from build123d import *

# Parameters (mm, degrees)
F0_R     = 10.16
F1_DEPTH = 76.2
F3_DEPTH = 27.94
F5_DEPTH = 10.16
F6_R     = 7.62
F7_DEPTH = 10.16
F8_R     = 10.16


with BuildPart() as f1:
    # F0 (on Front) → F1 (new body)
    with BuildSketch(Plane.XZ):
        Polygon((-96.203486, 15.24), (-96.203486, -20.32), (15.556514, -20.32), (51.116514, 15.24), (51.116514, 50.8), (15.556514, 50.8), (-20.003486, 15.24), align=None)
        Circle(F0_R, mode=Mode.SUBTRACT)
    extrude(amount=-F1_DEPTH)

    # F2 (on face) → F3 (cut)
    with BuildSketch(Plane.XY.offset(50.8)):
        with BuildLine():
            ThreePointArc((25.716514, 15.24), (33.336514, 7.62), (40.956514, 15.24))
            Line((40.956514, 15.24), (40.956514, 60.96))
            ThreePointArc((40.956514, 60.96), (33.336514, 68.58), (25.716514, 60.96))
            Line((25.716514, 60.96), (25.716514, 15.24))
        make_face()
    extrude(amount=-F3_DEPTH, mode=Mode.SUBTRACT)

    # F4 (on face) → F5 (cut)
    with BuildSketch(Plane.XY.offset(15.24)):
        with BuildLine():
            Line((-20.003486, 40.64), (-43.076643, 40.64))
            ThreePointArc((-43.076643, 40.64), (-58.103486, 53.34), (-73.130329, 40.64))
            Line((-73.130329, 40.64), (-96.203486, 40.64))
            Line((-96.203486, 40.64), (-96.203486, 35.56))
            Line((-96.203486, 35.56), (-73.130329, 35.56))
            ThreePointArc((-73.130329, 35.56), (-58.103486, 22.86), (-43.076643, 35.56))
            Line((-43.076643, 35.56), (-20.003486, 35.56))
            Line((-20.003486, 35.56), (-20.003486, 40.64))
        make_face()
    extrude(amount=-F5_DEPTH, mode=Mode.SUBTRACT)

    # F6 (on face) → F7 (cut)
    with BuildSketch(Plane.XY.offset(5.08)):
        with Locations((-58.103486, 38.1)):
            Circle(F6_R)
    extrude(amount=-F7_DEPTH, mode=Mode.SUBTRACT)

    # F8
    f8_edges = [f1.edges().sort_by_distance(p)[0] for p in [
        (-96.203486, 0, -2.54),
        (-96.203486, 76.2, -2.54),
    ]]
    fillet(f8_edges, radius=F8_R)


solid = f1.part
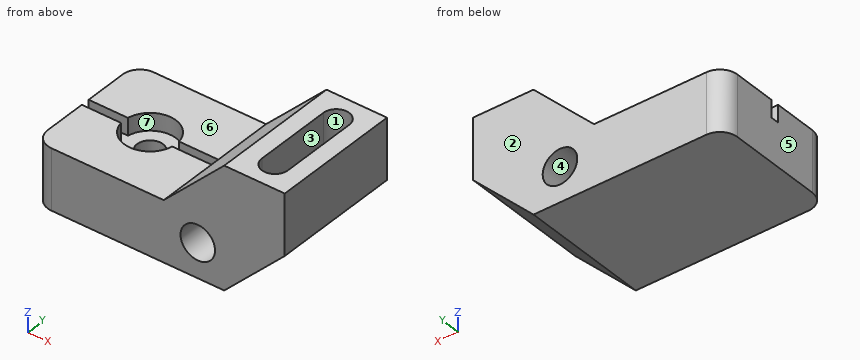
Could you check a few things on this model? Use its own coordinates, in mm. Face numbers are marked on the shaded views. A direction names the side the tool comes from. Give positions to 0.01 mm unless a question says otherwise; leave off trailing zeros. Order: outer loops, then holes, each group sorted by start corner. A loop starts at its lowest first (then second) coordinate and runs counter-clockwise, first axis right, second up. Notation, with made-up numbers: (1, -8.75) - (29, -8.75) arc R29 cw to (29, 21.25) - close; hole circle Ø5 at (57, 8.5). An arc over 180 degrees is marked (long way). One line per question, with ' | ' between items. Start each with the question number.
Item 1: I want a section at D-D on x = -23.5. Write out the boundary of the cut face in (y, z), then the cut area to 3 significant figures.
Item 2: I need wall thicknesses on probe 1 along X at (y, z) = (31.5, 8.5); probe 2 along Z at (x, y) = (-87, 6); probe 3 along Z at (x, y) = (-63, 32). Which ranges of each line are inside material? Lowest first, please. Write a range as [from, to].
Item 3: I want a section at C-C on y = 38.1. Write out the boundary of the cut face in (x, z).
Item 4: For the marked faces 5, 6 and 7, which set-ups out of +Z, -Z, +X, -X, +Y, -Y let a thin tool reach every point of the face, with its end or its side?
Item 5: I want a section at A-A on z = 0. Write out the boundary of the cut face in (x, y), then the cut area to 3 significant figures.
Item 6: I want a section at B-B on x = -8.5. Write out the boundary of the cut face in (y, z).
Item 7: Thinking about a two-plate mould opening in Y: for the marked faces 1, 2, 3 and 4, which applies, pulls with the +Y half, pulls with the -Y half, needs draft (parallel to the pull), parting line crosses it, or undercut?
Item 8: I'm going to push flat-ended pins straight in: pin 1 Ø2 at (x, y) = (-80, 29) entering from +Z; pin 2 Ø7.5 at (x, y) = (33.5, 42) entering from +Z; pin 3 Ø4 at (y, z) = (38, 9) entering from -X. Where does each tip first touch, or does it pass through?
Verdict:
1) outline: (0, -20.32) - (76.2, -20.32) - (76.2, 15.24) - (40.64, 15.24) - (40.64, 5.08) - (35.56, 5.08) - (35.56, 15.24) - (0, 15.24) - close | area: 2,660 mm^2
2) probe 1: [-96.2, -71.84], [-44.37, -5.57], [5.57, 44.38] | probe 2: [-20.32, 15.24] | probe 3: [-20.32, 5.08]
3) outline: (-96.2, -20.32) - (15.56, -20.32) - (51.12, 15.24) - (51.12, 50.8) - (40.96, 50.8) - (40.96, 22.86) - (25.72, 22.86) - (25.72, 50.8) - (15.56, 50.8) - (-20, 15.24) - (-20, 5.08) - (-50.48, 5.08) - (-50.48, -5.08) - (-65.72, -5.08) - (-65.72, 5.08) - (-96.2, 5.08) - close; hole circle Ø20.32 at (0, 0)
4) face 5: +Z, -Z, -X, +Y, -Y | face 6: +Z, -X, +Y, -Y | face 7: +Z
5) outline: (-96.2, 10.16) arc R10.16 ccw to (-86.04, 0) - (-10.16, 0) - (-10.16, 76.2) - (-86.04, 76.2) arc R10.16 ccw to (-96.2, 66.04) - close; (10.16, 0) - (35.88, 0) - (35.88, 76.2) - (10.16, 76.2) - close; hole circle Ø15.24 at (-58.1, 38.1) | area: 8,290 mm^2
6) outline: (0, -20.32) - (76.2, -20.32) - (76.2, -5.57) - (0, -5.57) - close; (0, 5.57) - (76.2, 5.57) - (76.2, 26.74) - (0, 26.74) - close
7) face 1: undercut | face 2: pulls with the +Y half | face 3: undercut | face 4: needs draft
8) pin 1: z = 15.24 | pin 2: z = 22.86 | pin 3: x = -20
